For this review, use the dimensioned drawing (mm, ordinates from the lowest corner) and the shaded views. A direction names the side the tool comes from. Round coordinates to 2 decimals unless told otherwise and drop trailing zeros. Order: outer loops, then holes, each group sorted by start corner. A loop starts at its lowest first (then second) coordinate and runs counter-clockwise, first axis right, second up. Notation, with made-up numbers: (56.5, -11.75) - (86.5, -11.75) arc R17 ccw to (86.5, 13.25) - close; hole circle Ø9 at (-5, -5). An arc over 180 degrees is marked (long way). Write item = value, one per line.
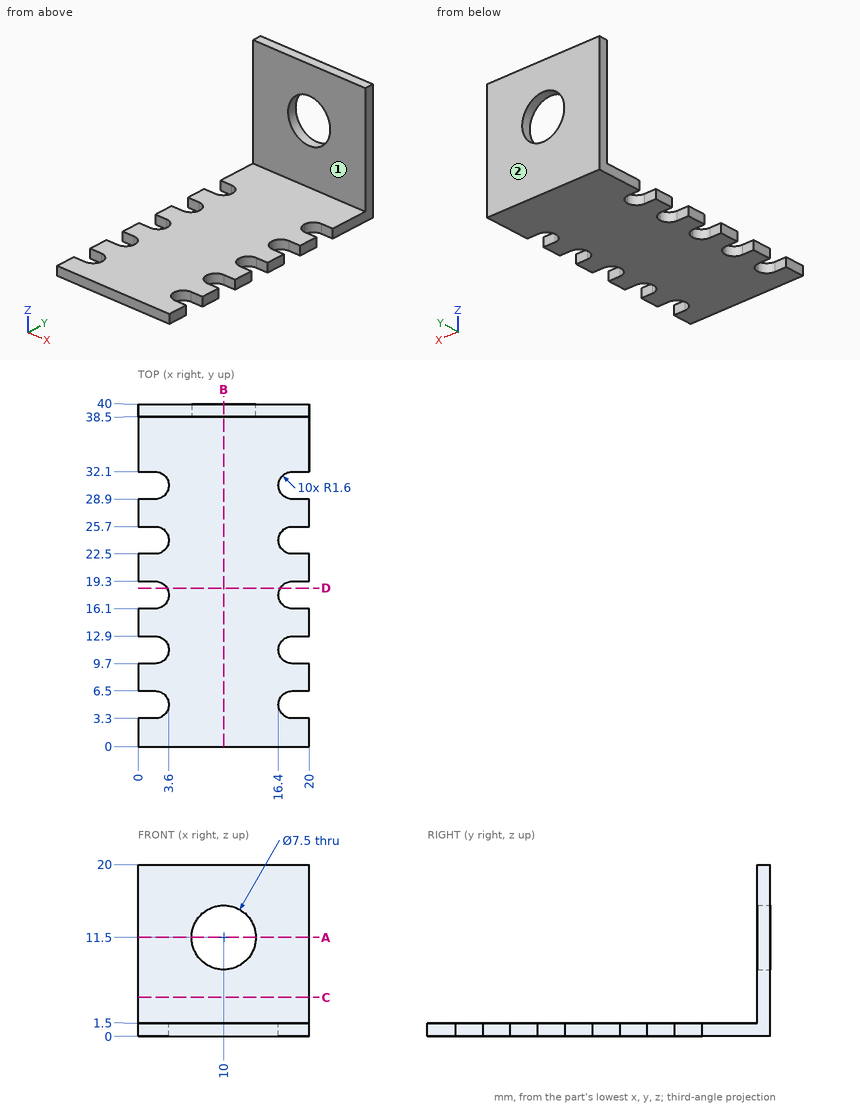
Item 1: Take a section at A-A, the plane z = 11.5. State the section outline as (x, y) points.
Data:
outline = (0, 38.5) - (6.25, 38.5) - (6.25, 40) - (0, 40) - close; (13.75, 38.5) - (20, 38.5) - (20, 40) - (13.75, 40) - close
Item 2: For line 1 along Z through (x, y) = (10, 39.2); line 2 along Y through (x, z) = (18, 6); line 3 along Z through (x, y) = (12.75, 16), list the stretches that pass through material, from the lowest coordinate up. Write a range as [from, to].
Data:
line_1 = [0, 7.75], [15.25, 20]
line_2 = [38.5, 40]
line_3 = [0, 1.5]
Item 3: Take a section at C-C, the plane z = 4.5. State the section outline as (x, y) points.
Data:
outline = (0, 38.5) - (20, 38.5) - (20, 40) - (0, 40) - close
Item 4: For the marked faces 1 and 2, list the 3-axis set-ups (+Z, -Z, +X, -X, +Y, -Y) from which the entire face can be reached by the end or side of a thin tool; tool diameter is ignored.
Data:
face_1 = +Z, +X, -X, -Y
face_2 = +Z, -Z, +X, -X, +Y
Item 5: Insertion check: P1, Ø2, axis at x = 4, z = 9.5, coming from the -Y side; P2, Ø1.5, axis at y = 33.5, z = 3, coming from the -X side; P3, Ø10, axis at x = 11, y = 14, coming from the +Z side. Each pin has a flat end and moves straight along its axis. Give the tip position at first contact, or say it passes through.
Data:
P1 = 38.5
P2 = through
P3 = 1.5
Item 6: Take a section at D-D, the plane y = 18.5. State the section outline as (x, z) points, and give its area (3 significant figures).
Data:
outline = (3.39, 0) - (16.61, 0) - (16.61, 1.5) - (3.39, 1.5) - close
area = 19.8 mm2
Item 7: Take a section at B-B, the plane x = 10. State the section outline as (y, z) points, and give its area (3 significant figures).
Data:
outline = (0, 0) - (40, 0) - (40, 7.75) - (38.5, 7.75) - (38.5, 1.5) - (0, 1.5) - close; (38.5, 15.25) - (40, 15.25) - (40, 20) - (38.5, 20) - close
area = 76.5 mm2
